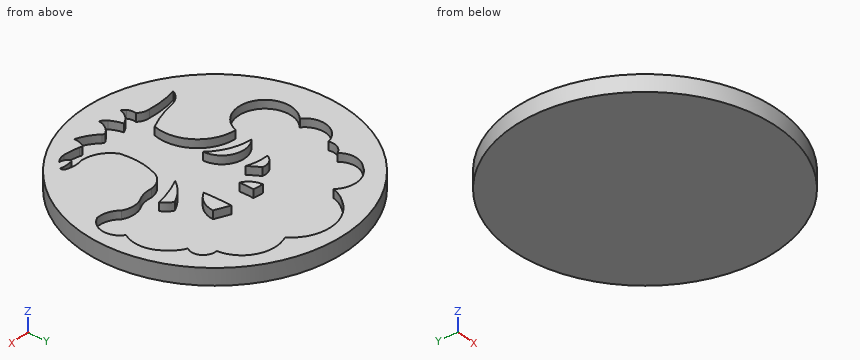
```python
from build123d import *

# Parameters (mm, degrees)
F0_R     = 50.8
F1_DEPTH = 6.35
F3_DEPTH = 3.175


with BuildPart() as f1:
    # F0 (on Top) → F1 (new body)
    with BuildSketch(Plane.XY):
        Circle(F0_R)
    extrude(amount=F1_DEPTH)

    # F2 (on face) → F3 (cut)
    with BuildSketch(Plane.XY.offset(6.35)):
        with BuildLine():
            ThreePointArc((-20.409899, -9.165186), (-8.713511, -15.533016), (-6.405892, -28.649023))
            ThreePointArc((-6.405892, -28.649023), (-12.498571, -30.92391), (-18.853704, -32.30527))
            ThreePointArc((-18.853704, -32.30527), (-21.972675, -33.680035), (-24.105206, -36.339033))
            ThreePointArc((-24.105206, -36.339033), (-18.309615, -35.54218), (-12.460569, -35.654053))
            ThreePointArc((-12.460569, -35.654053), (-10.157818, -36.115918), (-8.238821, -37.469961))
            ThreePointArc((-8.238821, -37.469961), (-8.312029, -39.074644), (-7.786276, -40.592521))
            ThreePointArc((-7.786276, -40.592521), (-7.173062, -41.29787), (-6.405892, -41.831724))
            ThreePointArc((-6.405892, -41.831724), (-4.778592, -38.642786), (-1.789923, -36.671672))
            ThreePointArc((-1.789923, -36.671672), (-1.085393, -39.0133), (0, -41.204534))
            ThreePointArc((0, -41.204534), (0.873752, -42.269552), (2.058734, -42.972066))
            ThreePointArc((2.058734, -42.972066), (3.026163, -40.087128), (5.10915, -37.869032))
            ThreePointArc((5.10915, -37.869032), (5.90739, -37.51004), (6.70563, -37.869032))
            ThreePointArc((6.70563, -37.869032), (10.017439, -40.631321), (13.8848, -42.539682))
            ThreePointArc((13.8848, -42.539682), (14.078165, -40.618723), (14.740057, -38.80506))
            ThreePointArc((14.740057, -38.80506), (15.40462, -38.390072), (16.165486, -38.577001))
            ThreePointArc((16.165486, -38.577001), (19.134333, -39.233369), (22.152284, -39.6033))
            ThreePointArc((22.152284, -39.6033), (24.22883, -39.250722), (26.057957, -38.20638))
            ThreePointArc((26.057957, -38.20638), (24.409477, -37.750926), (23.082776, -36.671672))
            ThreePointArc((23.082776, -36.671672), (23.305789, -35.851729), (24.132207, -35.654053))
            ThreePointArc((24.132207, -35.654053), (26.246167, -35.540671), (28.329933, -35.914309))
            ThreePointArc((28.329933, -35.914309), (28.305036, -34.988535), (27.65722, -34.32671))
            ThreePointArc((27.65722, -34.32671), (24.34987, -33.525294), (20.957004, -33.788539))
            ThreePointArc((20.957004, -33.788539), (15.180236, -31.980008), (11.14397, -27.468866))
            ThreePointArc((11.14397, -27.468866), (10.709627, -19.910276), (12.538101, -12.56333))
            ThreePointArc((12.538101, -12.56333), (15.245467, -9.599875), (19.090848, -8.448814))
            ThreePointArc((19.090848, -8.448814), (22.690074, -8.35066), (26.057957, -7.077309))
            ThreePointArc((26.057957, -7.077309), (29.897773, -6.621777), (33.567846, -7.839257))
            ThreePointArc((33.567846, -7.839257), (36.947302, -10.299215), (41.085728, -10.887046))
            ThreePointArc((41.085728, -10.887046), (45.507777, -5.155106), (42.558827, 1.456501))
            ThreePointArc((42.558827, 1.456501), (44.188538, 8.812407), (41.085728, 15.67811))
            ThreePointArc((41.085728, 15.67811), (38.938533, 18.174445), (36.168348, 19.954393))
            ThreePointArc((36.168348, 19.954393), (36.881996, 23.901454), (34.229763, 26.910482))
            ThreePointArc((34.229763, 26.910482), (33.036992, 27.313356), (31.778026, 27.309604))
            ThreePointArc((31.778026, 27.309604), (25.270382, 37.388286), (13.300548, 38.19596))
            ThreePointArc((13.300548, 38.19596), (0.47393, 45.12883), (-12.460569, 38.399376))
            ThreePointArc((-12.460569, 38.399376), (-14.182386, 35.784343), (-15.245431, 32.83935))
            ThreePointArc((-15.245431, 32.83935), (-22.776904, 35.86315), (-29.891349, 31.957883))
            ThreePointArc((-29.891349, 31.957883), (-32.28661, 26.905181), (-30.569399, 21.583691))
            ThreePointArc((-30.569399, 21.583691), (-33.136528, 19.1829), (-33.401847, 15.67811))
            ThreePointArc((-33.401847, 15.67811), (-39.802605, 9.763866), (-37.169039, 1.456501))
            ThreePointArc((-37.169039, 1.456501), (-35.724093, -14.795951), (-20.409899, -9.165186))
        make_face()
        with BuildLine():
            ThreePointArc((-19.671235, -2.408931), (-10.495474, -1.403019), (-5.499953, -9.165186))
            ThreePointArc((-5.499953, -9.165186), (-11.918937, -4.388742), (-19.671235, -2.408931))
        make_face(mode=Mode.SUBTRACT)
        with BuildLine():
            ThreePointArc((11.486482, -5.712907), (15.204523, -1.644017), (19.912776, 1.221651))
            ThreePointArc((19.912776, 1.221651), (21.825364, -0.176932), (23.082776, -2.185152))
            ThreePointArc((23.082776, -2.185152), (17.151026, -3.509855), (11.486482, -5.712907))
        make_face(mode=Mode.SUBTRACT)
        with BuildLine():
            ThreePointArc((-10.517537, 9.38917), (-9.26208, 7.248359), (-7.786276, 5.253054))
            ThreePointArc((-7.786276, 5.253054), (-11.891821, 6.399429), (-16.145367, 6.676962))
            ThreePointArc((-16.145367, 6.676962), (-13.865306, 9.140813), (-10.517537, 9.38917))
        make_face(mode=Mode.SUBTRACT)
        with BuildLine():
            ThreePointArc((0, 9.38917), (-2.69509, 11.815598), (-3.800875, 15.269336))
            ThreePointArc((-3.800875, 15.269336), (-1.893817, 15.079444), (0, 14.78553))
            ThreePointArc((0, 14.78553), (-0.095241, 12.08735), (0, 9.38917))
        make_face(mode=Mode.SUBTRACT)
        with BuildLine():
            ThreePointArc((10.79395, 4.70623), (10.615223, 9.986429), (10.673, 15.269336))
            ThreePointArc((10.673, 15.269336), (13.432832, 14.049362), (16.165486, 12.769669))
            ThreePointArc((16.165486, 12.769669), (14.580089, 8.004927), (10.79395, 4.70623))
        make_face(mode=Mode.SUBTRACT)
    extrude(amount=-F3_DEPTH, mode=Mode.SUBTRACT)


solid = f1.part
```
Could you check a few things on this model? Use its own coordinates, in mm. Give positions to 0.01 mm unless a question says otherwise; leave off trailing zeros. Order: outer loops, then holes, each group sorted by start corner. A loop starts at its lowest first (then second) coordinate and runs counter-clockwise, first axis right, second up.
Q1. Suppose I cut it at D-D, the plane y = 11. Write out the boundary of the cut face in (x, z) (3 decimals), and give its area (3 significant figures).
Q2. Suppose I cut it at B-B, the plane z = 5.25. Count the separate pieces of the cut face and the enclosed holes in it, and give its area (3 significant figures).
Q3. Suppose I cut it at A-A, the plane y = -4.5. Write out the boundary of the cut face in (x, z) (3 decimals), and give its area (3 significant figures).
Q4. If I drill on line 1 along X through (y, z) = (1, 5); line 2 along X through (y, z) = (5, 4.5); line 3 along X through (y, z) = (7, 5.5), over which ranges is the centre line in solid material (lowest first)?
Q5. I'm going to push flat-ended pins straight in: P1, Ø16.5, axis at x = -30.22, y = -6.12, coming from the +Z side (3 decimals); P2, Ø2, axis at y = 2, z = 3.5, coming from the -X side; P3, Ø2, axis at x = -9.5, z = 5.5, coming from the +Y side. Where does each tip first touch, or does it pass through?
Q6. Suppose I cut it at C-C, the plane y = 41.5. Write out the boundary of the cut face in (x, z) (3 decimals).
Solution:
1. outline: (-49.595, 0) - (49.595, 0) - (49.595, 6.35) - (43.752, 6.35) - (43.752, 3.175) - (15.9, 3.175) - (15.9, 6.35) - (10.608, 6.35) - (10.608, 3.175) - (-0.08, 3.175) - (-0.08, 6.35) - (-2.078, 6.35) - (-2.078, 3.175) - (-39.366, 3.175) - (-39.366, 6.35) - (-49.595, 6.35) - close
1. area: 389 mm2
2. separate pieces: 6
2. enclosed holes: 1
2. area: 3,780 mm2
3. outline: (-50.6, 0) - (50.6, 0) - (50.6, 6.35) - (45.555, 6.35) - (45.555, 3.175) - (14.288, 3.175) - (14.288, 6.35) - (12.384, 6.35) - (12.384, 3.175) - (-6.942, 3.175) - (-6.942, 6.35) - (-11.689, 6.35) - (-11.689, 3.175) - (-40.371, 3.175) - (-40.371, 6.35) - (-50.6, 6.35) - close
3. area: 391 mm2
4. line 1: x = -50.79 to -37.64, 19.41 to 20.34, 43.14 to 50.79
4. line 2: x = -50.55 to -39.62, 10.78 to 11.35, 43.97 to 50.55
4. line 3: x = -50.32 to -40.04, -16 to -9.1, 10.69 to 13.81, 44.24 to 50.32
5. P1: stops at z = 3.175
5. P2: stops at x = -50.79
5. P3: stops at y = 50.08
6. outline: (-29.298, 0) - (29.298, 0) - (29.298, 6.35) - (10.34, 6.35) - (10.34, 3.175) - (-9.637, 3.175) - (-9.637, 6.35) - (-29.298, 6.35) - close
